Here's how the part is built. I have some questions about the finished solid (model axes, mm). Give positions to 0.01 mm unless a question says otherwise; leave off trailing zeros. Write each loop counter-clockwise with the first axis right and the second up, starting at its lowest first coordinate (ties: lowest second). Pieces come first, ordered by that corner, then holes. Notation, with made-up numbers: (-25.5, 39.5) - (22.5, 39.5) arc R38 cw to (22.5, 77.5) - close; hole circle Ø4 at (82, 35). An arc over 180 degrees is marked (long way). One line per item, written item: value. Start each with the question number.
1) Imagine slicing it at C-C on z = 8. Write out the boundary of the cut face in (x, y).
2) Imagine slicing it at D-D on x = 15. Write out the boundary of the cut face in (y, z).
3) Imagine slicing it at A-A on y = 1.85. Write out the boundary of the cut face in (x, z), plus the area to 3 significant figures.
4) We'd pull the mould along Z, two halves only. Please class faces 1 (the cylindrical face through (-0.27, 1.23, 21.22)), 2 (the flat face through (17.752, 1.232, 7.949)), 3 (the cylindrical face through (34.842, 1.232, 24.494)): +Z half, -Z half, draft (parallel to the pull), parting line (faces both ways), or undercut.
5) Please list where these lines run through material, in increasing order: L1, parallel to Z at x = 0, y = 1.9; L2, parallel to Z at x = 0.5, y = 0.7; L3, parallel to X at y = 0.65, z = 0. Write a range as [from, to].
6) I'm going to push flat-ended pins straight in: P1, Ø2, axis at x = 0, z = 20, coming from the +Y side; P2, Ø1.5, axis at x = 16.5, y = 1, coming from the -Z side. Where does each tip first touch, or does it pass through?
7) Imagine slicing it at B-B on x = 0. Write out the boundary of the cut face in (y, z), plus the area to 3 significant figures.
from build123d import *

# Parameters (mm, degrees)
SKETCH1_R           = 1.25
BOSS_EXTRUDE1_DEPTH = 2.5


with BuildPart() as part:
    # Sketch1 → Boss-Extrude1 (new body)
    with BuildSketch(Plane(origin=(0, 0, 0), x_dir=(1, 0, 0), z_dir=(0, 1, 0))):
        with BuildLine():
            Line((2.542410714, 3.405678752), (33.393853524, -19.625571248))
            ThreePointArc((33.393853524, -19.625571248), (34.814441101, -24.566549497), (30.435868213, -27.260883288))
            Line((30.435868213, -27.260883288), (-0.415574597, -24.229633288))
            ThreePointArc((-0.415574597, -24.229633288), (-3.148705451, -22.85449715), (-4.25, -20))
            Line((-4.25, -20), (-4.25, 0))
            ThreePointArc((-4.25, 0), (-1.904895596, 3.7991937), (2.542410714, 3.405678752))
        make_face()
        Circle(SKETCH1_R, mode=Mode.SUBTRACT)
        with Locations((0, -20)):
            Circle(SKETCH1_R, mode=Mode.SUBTRACT)
        with Locations((30.85144281, -23.03125)):
            Circle(SKETCH1_R, mode=Mode.SUBTRACT)
    extrude(amount=BOSS_EXTRUDE1_DEPTH)


solid = part.part
Numbers:
1. outline: (-4.25, 0) - (17.82, 0) - (17.82, 2.5) - (-4.25, 2.5) - close
2. outline: (0, 5.89) - (2.5, 5.89) - (2.5, 25.74) - (0, 25.74) - close
3. outline: (-4.25, 0) arc R4.25 ccw to (2.54, -3.41) - (33.39, 19.63) arc R4.25 ccw to (30.44, 27.26) - (-0.42, 24.23) arc R4.25 ccw to (-4.25, 20) - close; hole circle Ø2.5 at (0, 0); hole circle Ø2.5 at (0, 20); hole circle Ø2.5 at (30.85, 23.03)
3. area: 731 mm^2
4. face 1: undercut
4. face 2: -Z half
4. face 3: parting line
5. L1: [-4.25, -1.25], [1.25, 18.75], [21.25, 24.27]
5. L2: [-4.22, -1.15], [1.15, 18.85], [21.15, 24.32]
5. L3: [-4.25, -1.25], [1.25, 7.1]
6. P1: through
6. P2: z = 6.45
7. outline: (0, -4.25) - (2.5, -4.25) - (2.5, -1.25) - (0, -1.25) - close; (0, 1.25) - (2.5, 1.25) - (2.5, 18.75) - (0, 18.75) - close; (0, 21.25) - (2.5, 21.25) - (2.5, 24.27) - (0, 24.27) - close
7. area: 58.8 mm^2
